For this review, use the dimensioned drawing (mm, ordinates from the lowest corner) and the shaded views. Round coordinates to 2 decimals unless told otherwise and drop trailing zeros. Order: outer loops, then holes, each group sorted by start corner. A loop starts at its lowest first (then second) coordinate and runs counter-clockwise, first axis right, second up. Notation, with made-up numbers: M 62.25,79 L 87.25,79 A9 ccw 87.25,88 Z; hole C 61,-26 d7. An arc over 180 degrees is marked long. Use a Markdown table: item, result. Add a question column.
1. The part is to be moulded in two halves that separate along Z. For the marked faces 1 and 2, say which applies: +Z half, -Z half, draft (parallel to the pull), parting line (faces both ways), or undercut.
2. Consider section A-A on x = 6. State the section outline as (y, z) points.
3. Consider section C-C on x = 1.5. State the section outline as (y, z) points.
4. To check wall thickness, follow probe 1 along Z at (x, y) = (8, 16.5) (1 decimal); probe 2 along X at (y, z) = (20, 32); probe 3 along Y at (x, z) = (2.5, 10). State the ranges of each line that lie inside material, in increasing order.
5. Consider section B-B on z = 10. State the section outline as (x, y) points, then the cut area to 4 significant figures.
6. Insertion check: P1, Ø3, axis at y = 13.5, z = 26.5, coming from the +X side; P2, Ø5, axis at y = 20, z = 70, coming from the -X side; P3, Ø1.5, axis at x = 7.5, z = 71, coming from the +Y side; P4, Ø4, axis at x = 7.5, z = 68.5, coming from the -Y side. Each pin has a flat end and moves straight along its axis. Give the tip position at first contact, or say it passes through.
7. Consider section D-D on z = 53.5. State the section outline as (x, y) points.
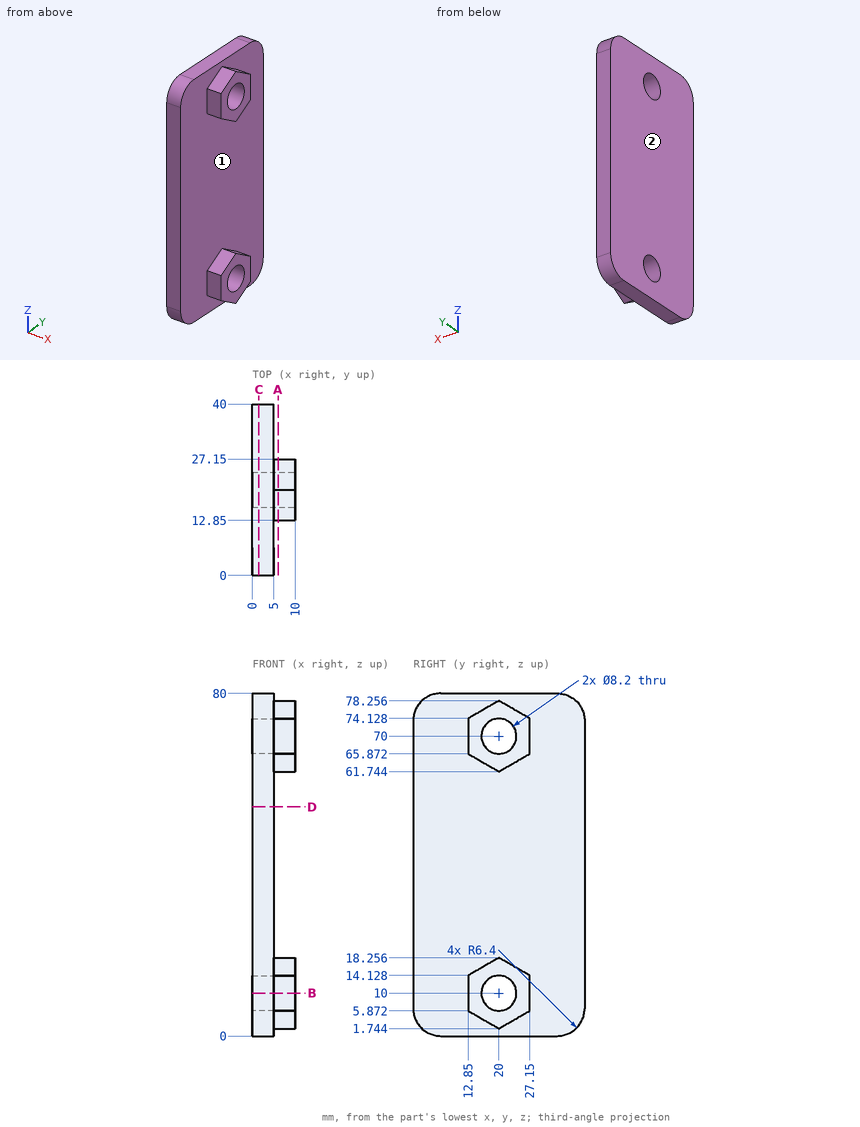
Answer block:
| question | item | result |
|---|---|---|
| 1 | face 1 | undercut |
| 1 | face 2 | draft |
| 2 | outline | M 12.85,5.87 L 20,1.74 L 27.15,5.87 L 27.15,14.13 L 20,18.26 L 12.85,14.13 Z; M 12.85,65.87 L 20,61.74 L 27.15,65.87 L 27.15,74.13 L 20,78.26 L 12.85,74.13 Z; hole C 20,10 d8.2; hole C 20,70 d8.2 |
| 3 | outline | M 0,6.4 A6.4 ccw 6.4,0 L 33.6,0 A6.4 ccw 40,6.4 L 40,73.6 A6.4 ccw 33.6,80 L 6.4,80 A6.4 ccw 0,73.6 Z; hole C 20,10 d8.2; hole C 20,70 d8.2 |
| 4 | probe 1 | 3.8 to 7.9, 12.1 to 16.2, 63.8 to 67.9, 72.1 to 76.2 |
| 4 | probe 2 | 0 to 5 |
| 4 | probe 3 | 0 to 15.9, 24.1 to 40 |
| 5 | outline | M 0,0 L 5,0 L 5,12.85 L 10,12.85 L 10,15.9 L 0,15.9 Z; M 0,24.1 L 10,24.1 L 10,27.15 L 5,27.15 L 5,40 L 0,40 Z |
| 5 | area | 189.5 mm^2 |
| 6 | P1 | x = 5 |
| 6 | P2 | through |
| 6 | P3 | y = 27.15 |
| 6 | P4 | y = 12.85 |
| 7 | outline | M 0,0 L 5,0 L 5,40 L 0,40 Z |
